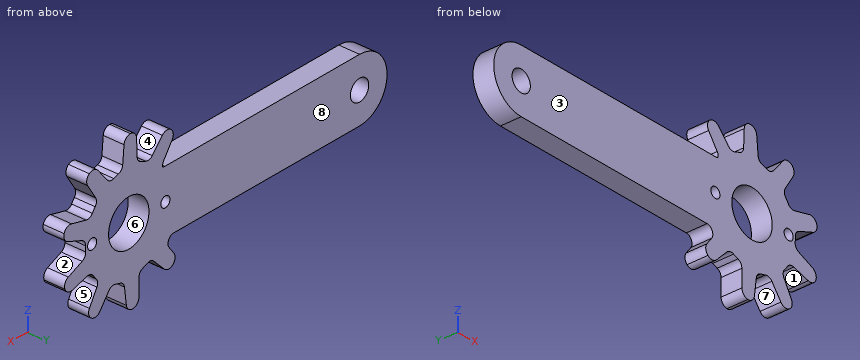
```python
from build123d import *

# Parameters (mm, degrees)
CROQUIS1_R              = 1.5875
SALIENTE_EXTRUIR1_DEPTH = 3.175
SALIENTE_EXTRUIR2_START = -3.175
CROQUIS2_R              = 7.5
CROQUIS2_R_2            = 1.5875
SALIENTE_EXTRUIR2_DEPTH = 3.175
CROQUIS7_R              = 3.5
CROQUIS7_R_2            = 0.79375
CORTAR_EXTRUIR3_DEPTH   = 10
SALIENTE_EXTRUIR3_START = -3.175
SALIENTE_EXTRUIR3_DEPTH = 3.175
CORTAR_EXTRUIR4_START   = -10
CORTAR_EXTRUIR4_DEPTH   = 10
MATRIZC1_COUNT          = 8
MATRIZC1_ANGLE          = 259
REDONDEO1_R             = 1


with BuildPart() as part:
    # Croquis1 → Saliente-Extruir1 (new body)
    with BuildSketch(Plane(origin=(0, 0, 0), x_dir=(1, 0, 0), z_dir=(0, 1, 0))):
        with BuildLine():
            Line((-20, 0), (20, 0))
            ThreePointArc((20, 0), (24.7625, -4.7625), (20, -9.525))
            Line((20, -9.525), (-20, -9.525))
            ThreePointArc((-20, -9.525), (-24.7625, -4.7625), (-20, 0))
        make_face()
        with Locations(Location((-20, -4.7625, 0), (0, 0, 270))):
            Circle(CROQUIS1_R, mode=Mode.SUBTRACT)
        with Locations(Location((20, -4.7625, 0), (0, 0, 270))):
            Circle(CROQUIS1_R, mode=Mode.SUBTRACT)
    extrude(amount=SALIENTE_EXTRUIR1_DEPTH)

    # Croquis2 → Saliente-Extruir2 (add)
    with BuildSketch(Plane(origin=(0, 3.175, 0), x_dir=(1, 0, 0), z_dir=(0, 1, 0)).offset(SALIENTE_EXTRUIR2_START)):
        with Locations((20, -4.7625)):
            Circle(CROQUIS2_R)
        with Locations(Location((20, -4.7625, 0), (0, 0, 270))):
            Circle(CROQUIS2_R_2, mode=Mode.SUBTRACT)
    extrude(amount=SALIENTE_EXTRUIR2_DEPTH)

    # Croquis7 → Cortar-Extruir3 (cut)
    with BuildSketch(Plane(origin=(0, 3.175, 0), x_dir=(1, 0, 0), z_dir=(0, 1, 0))):
        with Locations(Location((20, -4.7625, 0), (0, 0, 270))):
            Circle(CROQUIS7_R)
        with Locations(Location((13.65, -4.7625, 0), (0, 0, 270))):
            Circle(CROQUIS7_R_2)
        with Locations(Location((26.35, -4.7625, 0), (0, 0, 270))):
            Circle(CROQUIS7_R_2)
    extrude(amount=-CORTAR_EXTRUIR3_DEPTH, mode=Mode.SUBTRACT)

    # Croquis8 → Saliente-Extruir3 (add)
    with BuildSketch(Plane(origin=(0, 3.175, 0), x_dir=(1, 0, 0), z_dir=(0, 1, 0)).offset(SALIENTE_EXTRUIR3_START)):
        with BuildLine():
            Line((11.607813982, 3.461471902), (14.206158981, 0))
            ThreePointArc((14.206158981, 0), (15.121179891, 0.933736858), (16.184441281, 1.694396442))
            Line((16.184441281, 1.694396442), (13.163387879, 4.793819098))
            ThreePointArc((13.163387879, 4.793819098), (12.356515163, 4.161604411), (11.607813982, 3.461471902))
        make_face()
    saliente_extruir3 = extrude(amount=SALIENTE_EXTRUIR3_DEPTH)

    # Croquis9 → Cortar-Extruir4 (cut)
    with BuildSketch(Plane(origin=(0, 3.175, 0), x_dir=(1, 0, 0), z_dir=(0, 1, 0)).offset(CORTAR_EXTRUIR4_START)):
        with BuildLine():
            ThreePointArc((12.35651523, 4.161604469), (11.974526132, 3.819706546), (11.607813982, 3.461471902))
            Line((11.607813982, 3.461471902), (12.19397403, 2.680599255))
            ThreePointArc((12.19397403, 2.680599255), (11.982381708, 3.453243741), (12.35651523, 4.161604469))
        make_face()
        with BuildLine():
            ThreePointArc((13.163387879, 4.793819098), (12.753054069, 4.486514795), (12.35651523, 4.161604469))
            ThreePointArc((12.35651523, 4.161604469), (13.113956627, 4.422436237), (13.844906618, 4.094621057))
            Line((13.844906618, 4.094621057), (13.163387879, 4.793819098))
        make_face()
    cortar_extruir4 = extrude(amount=CORTAR_EXTRUIR4_DEPTH, mode=Mode.SUBTRACT)

    # MatrizC1: Saliente-Extruir3, Cortar-Extruir4 ×8 about axis
    matrizc1_axis = Axis((20, 0, 4.7625), (0, -1, 0))
    add([saliente_extruir3.rotate(matrizc1_axis, i * MATRIZC1_ANGLE / (MATRIZC1_COUNT - 1)) for i in range(1, MATRIZC1_COUNT)])
    add([cortar_extruir4.rotate(matrizc1_axis, i * MATRIZC1_ANGLE / (MATRIZC1_COUNT - 1)) for i in range(1, MATRIZC1_COUNT)], mode=Mode.SUBTRACT)

    # Redondeo1
    # the kernel refuses this fillet: 1 mm, written as the material it adds along each edge
    with BuildSketch(Plane(origin=(25.155056708, 0, -0.685012307), x_dir=(0.6933697506528057, 0, 0.7205819792915072), z_dir=(0, 1, 0)), Plane(origin=(27.395406089, 0, 3.514313802), x_dir=(0.12009264391370789, 0, 0.9927626891044079), z_dir=(0, 1, 0)), Plane(origin=(26.657411119, 0, 8.216320666), x_dir=(-0.501549250802915, 0, 0.8651290938461349), z_dir=(0, 1, 0)), Plane(origin=(23.238283761, 0, 11.527373856), x_dir=(-0.9212027273713431, 0, 0.389082941136718), z_dir=(0, 1, 0)), Plane(origin=(18.515005687, 0, 12.114016299), x_dir=(-0.9698611692594302, 0, -0.243658187555294), z_dir=(0, 1, 0)), Plane(origin=(14.389777858, 0, 9.739990082), x_dir=(-0.6279284118017822, 0, -0.7782711029275668), z_dir=(0, 1, 0)), Plane(origin=(16.184441281, 0, -1.694396442), x_dir=(0.8837864601497757, 0, -0.4678904710035554), z_dir=(0, 1, 0)), Plane(origin=(20.838616598, 0, -2.690467342), x_dir=(0.9874067650142349, 0, 0.15820202402031353), z_dir=(0, 1, 0))) as redondeo1_piece_1:
        with BuildLine():
            CenterArc((0.748840141, 0.998904162), REDONDEO1_R, 196.368950511, 70.948483307)
            Line((-0.210626698, 0.717082614), (0, 0))
            ThreePointArc((0, 0), (0.351018816, 0.008218784), (0.702037632, 0))
        make_face()
    extrude(amount=3.175)
    with BuildSketch(Plane(origin=(22.981009808, 0, -2.119620351), x_dir=(0.6032966406304949, 0, -0.7975168734289948), z_dir=(0, 1, 0)), Plane(origin=(26.522503707, 0, 1.06021079), x_dir=(0.9617717559465732, 0, -0.2738523132336944), z_dir=(0, 1, 0)), Plane(origin=(27.437196341, 0, 5.731061088), x_dir=(0.9329135130884484, 0, 0.36010050971495355), z_dir=(0, 1, 0)), Plane(origin=(25.35671448, 0, 10.011843767), x_dir=(0.5283439627642348, 0, 0.8490304217226758), z_dir=(0, 1, 0)), Plane(origin=(21.11892846, 0, 12.178563585), x_dir=(-0.0890050127232042, 0, 0.9960311780813601), z_dir=(0, 1, 0)), Plane(origin=(16.430517523, 0, 11.358619681), x_dir=(-0.6705090902301596, 0, 0.7419013141373477), z_dir=(0, 1, 0)), Plane(origin=(18.238976871, 0, -2.527822183), x_dir=(0.0018564846529317855, 0, -0.9999982767308818), z_dir=(0, 1, 0))) as redondeo1_piece_2:
        with BuildLine():
            CenterArc((0.747376131, 1), REDONDEO1_R, 199.051516693, 70.948483307)
            ThreePointArc((-0.197849332, 0.673581828), (-0.091039016, 0.339107144), (0, 0))
            Line((0, 0), (0.747376131, 0))
        make_face()
    extrude(amount=3.175)
    with BuildSketch(Plane(origin=(14.206158981, 3.175, 0), x_dir=(-1, 0, 0), z_dir=(0, -1, 0))) as redondeo1_piece_3:
        with BuildLine():
            CenterArc((REDONDEO1_R * 2.00103600097, REDONDEO1_R), REDONDEO1_R, 143.106368796, 126.893631204)
            Line((REDONDEO1_R * 1.20128460683, REDONDEO1_R * 1.6003313315), (0, 0))
            Line((0, 0), (REDONDEO1_R * 2.00103600097, 0))
        make_face()
    extrude(amount=3.175)
    with BuildSketch(Plane(origin=(14.206158981, 3.175, 9.525), x_dir=(-1, 0, 0), z_dir=(0, -1, 0))) as redondeo1_piece_4:
        with BuildLine():
            CenterArc((0.454646298, -1), REDONDEO1_R, 90, 47.317031956)
            ThreePointArc((-0.280469857, -0.322058824), (-0.137942125, -0.163026135), (0, 0))
            Line((0, 0), (0.454646298, 0))
        make_face()
    extrude(amount=3.175)


solid = part.part
```
The listing builds one solid part. Answer for the finished solid, in the listing's coordinates (mm). Face numbers are marked on the shaded views. A direction names the side the tool comes from. Coordinates: 2 decimals unless noted, no trailing zeros. Answer as CSV lines item,"result". Start each with the question number.
(1) The part is cut by section A-A (y = 0.7). State how many separate pieces and enclosed holes the cut face has, and give its area (3 significant figures).
(2) Given pin 1 (12 mm diameter, centred on x = -9, z = 1, fed in from -Y); pin 2 (1 mm diameter, centred on x = -6.5, y = 1.5, fed in from +Z) (3 decimals); pin 3 (1 mm diameter, centred on y = 1, z = 1, fed in from -X); pin 4 (1 mm diameter, centred on x = -17, y = 2, fed in from -Z), each flat-ended and moving along its own axis, determine where each tip first touches the part or whether it passes through.
(3) The mould has two halves that part along Z. Classify the marked faces 5, 6, 7 and 8: pulls with the +Z half, pulls with the -Z half, needs draft (parallel to the pull), parting line crosses it, or undercut.
(4) For the marked faces 1, 2, 3 and 4, determine the directions among +Z, -Z, +X, -X, +Y, -Y from which every point of the face is accessible in a straight line to the end or side of a thin tool.
(5) Find the intervals of material crossed by L1, parallel to Z at x = 10.5, y = 1.25 (3 decimals); L2, parallel to X at y = 0.9, z = 10; L3, parallel to X at y = 3.05, z = 14.25, in increasing order. Write a range as [from, to].
Determined:
1,separate pieces,"1"
1,enclosed holes,"4"
1,area,"555 mm2"
2,pin 1,"y = 0"
2,pin 2,"z = 9.525"
2,pin 3,"x = -23.47"
2,pin 4,"z = 0"
3,face 5,"undercut"
3,face 6,"undercut"
3,face 7,"pulls with the -Z half"
3,face 8,"needs draft"
4,face 1,"-Z, +Y, -Y"
4,face 2,"+X, +Y, -Y"
4,face 3,"+Z, -Z, +X, -X, -Y"
4,face 4,"+Z, +Y, -Y"
5,L1,"[0, 9.525]"
5,L2,"[14.12, 25.61]"
5,L3,"[18.6, 20.93], [25.48, 26.92]"
